Autodesk Inventor part; units mm, degrees
ref_plane "YZ Plane" through (0, 0, 0) normal (1, 0, 0) x (0, 1, 0)
ref_plane "XZ Plane" through (0, 0, 0) normal (0, 1, 0) x (-1, 0, 0)
ref_plane "XY Plane" through (0, 0, 0) normal (0, 0, 1) x (1, 0, 0)
ref_plane "Work Plane2" through (0, 0, -27.25) normal (1, 0, 0) x (0, 1, 0)
sketch "Sketch5" plane through (0, 0, -27.25) normal (1, 0, 0) x (0, 1, 0)
  circle A0 centre (10.1974, 36.4793) radius 2.25
  circle A1 centre (12.5, 27.25) radius 2.25
  circle A2 centre (9.8332, 17.5326) radius 2.25
  circle A3 centre (4.5689, 39.8851) radius 2.25
  circle A4 centre (3.4977, 14.2493) radius 2.25
  circle A5 centre (-4.5689, 16.6149) radius 2.25
  circle A6 centre (-10.1974, 22.0207) radius 2.25
  circle A7 centre (-12.5, 27.25) radius 2.25
  circle A8 centre (-9.8332, 32.9674) radius 2.25
  circle A9 centre (-3.4977, 38.2507) radius 2.25
  circle A10 centre (0, 27.25) radius 25.4
  circle A11 centre (0, 27.25) radius 8.255
  dimension "d16" = 50.8
  dimension "d17" = 16.51
extrude "Extrusion3" add sketch "Sketch5" along normal blind 1.27
sketch "Sketch6" plane through (1.27, 0, 0) normal (1, 0, 0) x (0, 0, -1)
  line L0 (-35.56, 0) -> (35.56, 0)
  line L1 (0, -35.56) -> (0, 35.56)
  circle A0 centre (0, 0) radius 19.05
  circle A1 centre (0, 0) radius 22.225
  point P0 (0, 0)
  dimension "d20" = 38.1
  dimension "d21" = 3.175
extrude "Extrusion4" add sketch "Sketch6" along normal blind 25.4 contours A0 L1 A1 L0 | L0 A1 L1 A0 | A0 L0 A1 L1 | L1 A1 L0 A0
sketch "Sketch9" plane through (26.67, 0, 0) normal (1, 0, 0) x (0, 0, -1)
  line L0 (35.56, 0) -> (-35.56, 0)
  line L1 (0, 0) -> (6.5155, 17.9011) construction
  circle A0 centre (0, 0) radius 22.225 construction
  line L2 (0, 0) -> (6.5155, -17.9011) construction
  arc A1 (7.6014, -20.8847) -> (7.6014, 20.8847) centre (0, 0) ccw
  circle A2 centre (0, 0) radius 19.05 construction
  arc A3 (6.5155, -17.9011) -> (6.5155, 17.9011) centre (0, 0) ccw
  line L3 (6.5155, 17.9011) -> (7.6014, 20.8847)
  line L4 (6.5155, -17.9011) -> (7.6014, -20.8847)
  dimension "d31" = 140
extrude "Extrusion7" cut sketch "Sketch9" against normal up to surface (25.4 mm away)
fillet "Fillet4" radius 3.175 1 edges at (26.67, 0, 22.225)
fillet "Fillet5" radius 3.175 3 edges at (1.27, 0, 22.225) (1.27, 19.3929, -7.0584) (1.27, -19.3929, -7.0584)
properties part number "PulleyCover" material "ABS Plastic"
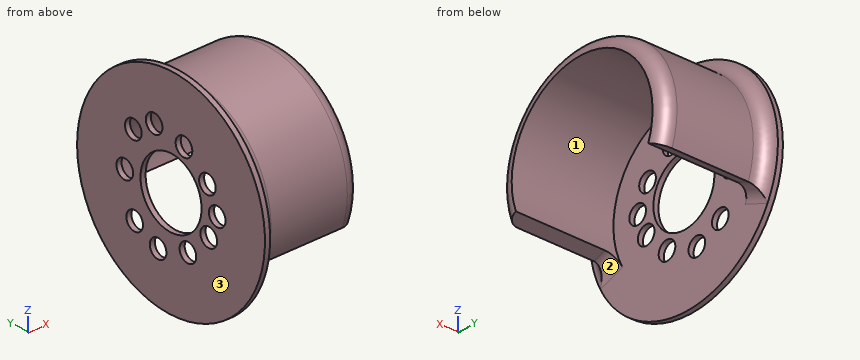
For this review, take the finished solid that the model builds, in its own axes (mm). Face numbers are marked on the shaded views. Give positions to 0.01 mm unless a question says otherwise; leave off trailing zeros. Order: outer loops, then holes, each group sorted by start corner. A loop starts at its lowest first (then second) coordinate and runs counter-clockwise, first axis right, second up.
1) Insertion check: pin 1 (6 mm diameter, centred on y = 4.57, z = 12.64, fed in from +X); pin 2 (4 mm diameter, centred on x = 21.5, z = 16, fed in from -Y); pin 3 (5 mm diameter, centred on y = -4.57, z = -10.64, fed in from -X); pin 4 (8 mm diameter, centred on x = 18.5, y = 7.5, fed in from -Z). Each pin has a flat end and moves straight along its axis. Give the tip position at first contact, or say it passes through.
2) The part is to be moulded in two halves that separate along Z. For the marked faces 1, 2 and 3, say which applies: released by +Z, released by -Z, zero draft, split by the parting line, or undercut.
3) Take a section at B-B (x = 8). Give the boundary of the cut face in (y, z) (3 decimals), then the cut area to 3 significant figures.
4) Wall thickness on line 1 (X direction, y = 1, z = 16); line 2 (Y direction, x = 10.5, z = 2.5); line 3 (Y direction, x = 10.5, z = 13): over which ranges is each line inside the solid? List them lowest first.
Derived:
1. pin 1: stops at x = 1.27
1. pin 2: stops at y = -17.26
1. pin 3: stops at x = 0
1. pin 4: stops at z = 15.19
2. face 1: undercut
2. face 2: released by -Z
2. face 3: zero draft
3. outline: (-20.885, -7.601) - (-17.901, -6.516) arc R19.05 cw (long way) to (17.901, -6.516) - (20.885, -7.601) arc R22.225 ccw (long way) to start
3. area: 252 mm2
4. line 1: x = 0 to 1.27
4. line 2: y = -22.08 to -18.89, 18.89 to 22.08
4. line 3: y = -18.03 to -13.92, 13.92 to 18.03
